from build123d import *

# Parameters (mm, degrees)
F2_R     = 13.5980918735
F3_DEPTH = 228.6


# Not quite as in the source:
# - a fillet or chamfer that OpenCascade refuses, or shapes differently, is made with other operations: its cross-section is extruded or revolved along the edge and cut away or added


with BuildPart() as f1:
    # F0 (on Front) → F1 (revolve)
    with BuildSketch(Plane.XZ):
        with BuildLine():
            Line((25.3469641268, 61.8318257093), (-12.7530358732, 61.8318257093))
            Line((-12.7530358732, 61.8318257093), (-12.7530358732, 52.5684214187))
            ThreePointArc((-12.7530358732, 52.5684214187), (-5.1330358732, 44.9484214187), (-12.7530358732, 37.3284214187))
            Line((-12.7530358732, 37.3284214187), (-12.7530358732, -13.4300431368))
            ThreePointArc((-12.7530358732, -13.4300431368), (-4.6335244682, -21.5495545417), (-12.7530358732, -29.6690659466))
            Line((-12.7530358732, -29.6690659466), (-12.7530358732, -39.7681742907))
            Line((-12.7530358732, -39.7681742907), (25.3469641268, -39.7681742907))
            Line((25.3469641268, -39.7681742907), (25.3469641268, 61.8318257093))
        make_face()
    revolve(axis=Axis((25.3469641268, 0, 11.0318257093), (0, 0, -1)))

    # F2 (on Front) → F3 (join)
    with BuildSketch(Plane.XZ):
        with Locations((24.8341448605, 11.9163831696)):
            Circle(F2_R)
    extrude(amount=F3_DEPTH)

    # F4: chamfer of 5.08 on 4 edges, made by hand

    # F4_s1 → F4_t2 (revolve, cut)
    with BuildSketch(Plane.XZ):
        Polygon((-7.6730358732, 61.8318257093), (-12.7530358732, 56.7518257093), (-12.7530358732, 61.8318257093), align=None)
    revolve(axis=Axis((25.3469641268, 0, 61.8318257093), (0, 0, -1)), mode=Mode.SUBTRACT)

    # F4_s3 → F4_t4 (revolve, cut)
    with BuildSketch(Plane.XZ):
        with BuildLine():
            Line((-9.6281385439, -29.0436510274), (-12.7530358732, -33.7323580503))
            Line((-12.7530358732, -33.7323580503), (-12.7530358732, -29.6690659466))
            ThreePointArc((-12.7530358732, -29.6690659466), (-11.0871747515, -29.4963383048), (-9.6281385439, -29.0436510274))
        make_face()
    revolve(axis=Axis((25.3469641268, 0, -29.6690659466), (0, 0, -1)), mode=Mode.SUBTRACT)

    # F4_s5 → F4_t6 (revolve, cut)
    with BuildSketch(Plane.XZ):
        Polygon((-12.7530358732, -34.6881742907), (-7.6730358732, -39.7681742907), (-12.7530358732, -39.7681742907), align=None)
    revolve(axis=Axis((25.3469641268, 0, -39.7681742907), (0, 0, -1)), mode=Mode.SUBTRACT)


solid = f1.part
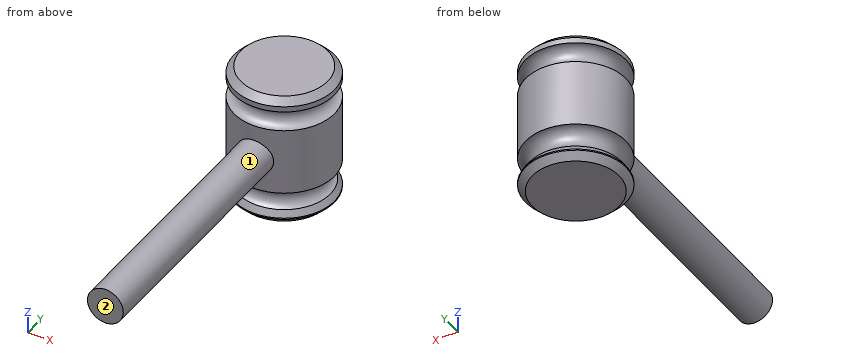
The listing builds one solid part. Answer for the finished solid, in the listing's coordinates (mm). Face numbers are marked on the shaded views. A direction names the side the tool comes from. Coordinates: 2 decimals unless noted, no trailing zeros. Loops run counter-clockwise (first coordinate to the right, second up) from the corner with the lowest first, then second, coordinate; pieces in that order, holes last. Notation, with made-up numbers: (28.25, 13) -> (35.25, 13) arc R24 ccw to (35.25, 37) -> close; hole circle Ø9 at (70, 14). An arc over 180 degrees is marked (long way). Answer in a Markdown table with one row per item. Add a question column.
1. Consider line 1 (Z direction, x = 25, y = -154); line 2 (Z direction, x = 26, y = -151.5); line 3 (X direction, y = -138, z = 20). Determine where each line is inside the solid, lowest interval first. Write a range as [from, to].
2. For the marked faces 1 and 2, determine the directions among +Z, -Z, +X, -X, +Y, -Y from which every point of the face is accessible in a straight line to the end or side of a thin tool.
3. Flat-ended cylindrical pins translate along their axes: P1, Ø4, axis at x = 20.5, y = -197.5, coming from the -Z side; P2, Ø10, axis at x = 27, z = 28, coming from the +Y side; P3, Ø8, axis at y = -186.5, z = 1.5, coming from the +X side. Find the tip coordinate at first contact, or state that the pin passes through.
4. The part is cut by section C-C, the plane y = -169. Write down the section's boundary in (x, z).
5. The part is cut by section A-A, the plane y = 0. Write down the section's boundary in (x, z).
6. The part is cut by section B-B, the plane z = 44. Write down the section's boundary in (x, y), then the cut area to 3 significant figures.
Answer below:
| question | item | result |
|---|---|---|
| 1 | line 1 | [-1.68, 25.51] |
| 1 | line 2 | [-1.63, 25.46] |
| 1 | line 3 | [13.9, 35.77] |
| 2 | face 1 | -Y |
| 2 | face 2 | +Z, -Z, +X, -X, -Y |
| 3 | P1 | z = -1.48 |
| 3 | P2 | y = 38.1 |
| 3 | P3 | x = 36.82 |
| 4 | outline | circle Ø27.2 at (24.83, 11.92) |
| 5 | outline | (-12.75, -34.69) -> (-7.67, -39.77) -> (58.37, -39.77) -> (63.45, -34.69) -> (63.45, -33.73) -> (60.32, -29.04) arc R8.12 cw to (63.45, -13.43) -> (63.45, 37.33) arc R7.62 cw to (63.45, 52.57) -> (63.45, 56.75) -> (58.37, 61.83) -> (-7.67, 61.83) -> (-12.75, 56.75) -> (-12.75, 52.57) arc R7.62 cw to (-12.75, 37.33) -> (-12.75, -13.43) arc R8.12 cw to (-9.63, -29.04) -> (-12.75, -33.73) -> close |
| 6 | outline | circle Ø61.08 at (25.35, 0) |
| 6 | area | 2,930 mm2 |
